Verification items for the finished model (mm, model axes). A direction names the side the tool comes from. Give positions to 0.01 mm unless a question says otherwise; leave off trailing zeros. Write each loop counter-clockwise with the first axis right and the second up, starting at its lowest first coordinate (ties: lowest second). Pieces come first, ordered by that corner, then holes. Notation, with made-up numbers: M 45.5,-15 L 62.5,-15 A16 ccw 62.5,-8 Z; hole C -21.75,84 d8. An arc over 180 degrees is marked long. Answer as a JSON object with one key per item and string values.
```python
from build123d import *

# Parameters (mm, degrees)
SKETCH_1_W        = 96
SKETCH_1_H        = 96
EXTRUDE_1_DEPTH   = 5.4
SKETCH_2_W        = 14
SKETCH_2_H        = 14
EXTRUDE_2_DEPTH   = 2.6
SKETCH_4_W        = 90
SKETCH_4_H        = 90
SKETCH_4_W_2      = 87
SKETCH_4_H_2      = 87
EXTRUDE_1_2_DEPTH = 1
SKETCH_5_R        = 1.5
EXTRUDE_3_DEPTH   = 14


with BuildPart() as part:
    # Эскиз1 → Extrude 1 (new body)
    with BuildSketch(Plane(origin=(0, 0, 0), x_dir=(1, 0, 0), z_dir=(0, 1, 0))):
        with Locations((6.473253846, 2.11160233)):
            Rectangle(SKETCH_1_W, SKETCH_1_H)
    extrude(amount=EXTRUDE_1_DEPTH)

    # Эскиз2 → Бобышка-Вытянуть2 (add)
    with BuildSketch(Plane(origin=(0, 5.4, 0), x_dir=(1, 0, 0), z_dir=(0, 1, 0))):
        with Locations((-3.026746154, 34.11160233)):
            Rectangle(SKETCH_2_W, SKETCH_2_H)
        with Locations((-22.026746154, 34.11160233)):
            Rectangle(SKETCH_2_W, SKETCH_2_H)
        with Locations((15.973253846, 34.11160233)):
            Rectangle(SKETCH_2_W, SKETCH_2_H)
        with Locations((34.973253846, 34.11160233)):
            Rectangle(SKETCH_2_W, SKETCH_2_H)
        with Locations((-3.026746154, 15.11160233)):
            Rectangle(SKETCH_2_W, SKETCH_2_H)
        with Locations((-22.026746154, 15.11160233)):
            Rectangle(SKETCH_2_W, SKETCH_2_H)
        with Locations((15.973253846, 15.11160233)):
            Rectangle(SKETCH_2_W, SKETCH_2_H)
        with Locations((34.973253846, 15.11160233)):
            Rectangle(SKETCH_2_W, SKETCH_2_H)
        with Locations((-3.026746154, -3.88839767)):
            Rectangle(SKETCH_2_W, SKETCH_2_H)
        with Locations((-22.026746154, -3.88839767)):
            Rectangle(SKETCH_2_W, SKETCH_2_H)
        with Locations((15.973253846, -3.88839767)):
            Rectangle(SKETCH_2_W, SKETCH_2_H)
        with Locations((34.973253846, -3.88839767)):
            Rectangle(SKETCH_2_W, SKETCH_2_H)
        with Locations((-3.026746154, -22.88839767)):
            Rectangle(SKETCH_2_W, SKETCH_2_H)
        with Locations((-22.026746154, -22.88839767)):
            Rectangle(SKETCH_2_W, SKETCH_2_H)
        with Locations((15.973253846, -22.88839767)):
            Rectangle(SKETCH_2_W, SKETCH_2_H)
        with Locations((34.973253846, -22.88839767)):
            Rectangle(SKETCH_2_W, SKETCH_2_H)
    extrude(amount=EXTRUDE_2_DEPTH)

    # Эскиз4 → Extrude 1 2 (add)
    with BuildSketch(Plane(origin=(0, 5.4, 0), x_dir=(1, 0, 0), z_dir=(0, 1, 0))):
        with Locations((6.473253846, 2.11160233)):
            Rectangle(SKETCH_4_W, SKETCH_4_H)
        with Locations((6.473253846, 2.11160233)):
            Rectangle(SKETCH_4_W_2, SKETCH_4_H_2, mode=Mode.SUBTRACT)
    extrude(amount=EXTRUDE_1_2_DEPTH)

    # Эскиз5 → Бобышка-Вытянуть3 (add)
    with BuildSketch(Plane.XZ):
        with Locations(Location((39.473253846, 25.88839767, 0), (0, 0, 90))):
            Circle(SKETCH_5_R)
        with Locations(Location((-26.526746154, 25.88839767, 0), (0, 0, 90))):
            Circle(SKETCH_5_R)
        with Locations(Location((-26.526746154, -30.11160233, 0), (0, 0, 90))):
            Circle(SKETCH_5_R)
        with Locations(Location((39.473253846, -30.11160233, 0), (0, 0, 90))):
            Circle(SKETCH_5_R)
    extrude(amount=EXTRUDE_3_DEPTH)


solid = part.part
```
1) Section check A-A on x = 35. Record the boundary of the cut face in (y, z).
Completed:
{"outline": "M 0,-50.11 L 5.4,-50.11 L 5.4,-47.11 L 6.4,-47.11 L 6.4,-45.61 L 5.4,-45.61 L 5.4,-41.11 L 8,-41.11 L 8,-27.11 L 5.4,-27.11 L 5.4,-22.11 L 8,-22.11 L 8,-8.11 L 5.4,-8.11 L 5.4,-3.11 L 8,-3.11 L 8,10.89 L 5.4,10.89 L 5.4,15.89 L 8,15.89 L 8,29.89 L 5.4,29.89 L 5.4,41.39 L 6.4,41.39 L 6.4,42.89 L 5.4,42.89 L 5.4,45.89 L 0,45.89 Z"}
2) Section check C-C on y = -5. Record the boundary of the cut face in (x, z), and give its area (3 significant figures).
Completed:
{"outline": "C -26.53,-30.11 d3; C -26.53,25.89 d3; C 39.47,-30.11 d3; C 39.47,25.89 d3", "area": "28.3 mm2"}
3) Section check B-B on z = 13. Record the boundary of the cut face in (x, y).
Completed:
{"outline": "M -41.53,0 L 54.47,0 L 54.47,5.4 L 51.47,5.4 L 51.47,6.4 L 49.97,6.4 L 49.97,5.4 L -37.03,5.4 L -37.03,6.4 L -38.53,6.4 L -38.53,5.4 L -41.53,5.4 Z"}
4) Thickness scan on L1, parallel to X at y = 5.75, z = -18; L2, parallel to X at y = 6.75, z = -31.5; L3, parallel to Z at x = 33, y = 6.25. Record the ranges inside material, lowest first.
Completed:
{"L1": "x = -38.53 to -37.03, -29.03 to -15.03, -10.03 to 3.97, 8.97 to 22.97, 27.97 to 41.97, 49.97 to 51.47", "L2": "x = -29.03 to -15.03, -10.03 to 3.97, 8.97 to 22.97, 27.97 to 41.97", "L3": "z = -47.11 to -45.61, -41.11 to -27.11, -22.11 to -8.11, -3.11 to 10.89, 15.89 to 29.89, 41.39 to 42.89"}
5) Release check for a two-part mould opening along X. For faces 3 (the face through (3, 5.4, 44)), 4 (the face through (39.02, -6.9, 27.32)), 5 (the face through (41.973, 7, -34)) record: pulls with the +X half, pulls with the -X half, needs draft (parallel to the pull), parting line crosses it, or undercut.
Completed:
{"face 3": "needs draft", "face 4": "undercut", "face 5": "undercut"}
6) Section check D-D on z = -36. Record the boundary of the cut face in (x, y).
Completed:
{"outline": "M -41.53,0 L 54.47,0 L 54.47,5.4 L 51.47,5.4 L 51.47,6.4 L 49.97,6.4 L 49.97,5.4 L 41.97,5.4 L 41.97,8 L 27.97,8 L 27.97,5.4 L 22.97,5.4 L 22.97,8 L 8.97,8 L 8.97,5.4 L 3.97,5.4 L 3.97,8 L -10.03,8 L -10.03,5.4 L -15.03,5.4 L -15.03,8 L -29.03,8 L -29.03,5.4 L -37.03,5.4 L -37.03,6.4 L -38.53,6.4 L -38.53,5.4 L -41.53,5.4 Z"}
7) Access from +Z, -Z, +X, -X, +Y, -Y to the whole of each face (thin tool, end or side, straight path). Record for faces 1 (the face through (3.973, 7, -34)), 2 (the face through (-22, 8, -34)).
Completed:
{"face 1": "+Y", "face 2": "+Z, -Z, +X, -X, +Y"}
8) Go/stop test with flat-tipped pins: pin 1 (1 mm diameter, centred on x = 0, z = -6.5, fed in from -Y); pin 2 (1.3 mm diameter, centred on y = 6.5, z = 22, fed in from -X); pin 3 (2 mm diameter, centred on x = -2, y = 6.5, fed in from -Z); pin 4 (1 mm diameter, centred on y = -1.5, z = 34.5, fed in from -X). Record where each tip stops, or that it passes through.
Completed:
{"pin 1": "stops at y = 0", "pin 2": "stops at x = -38.53", "pin 3": "stops at z = -47.11", "pin 4": "passes through"}
